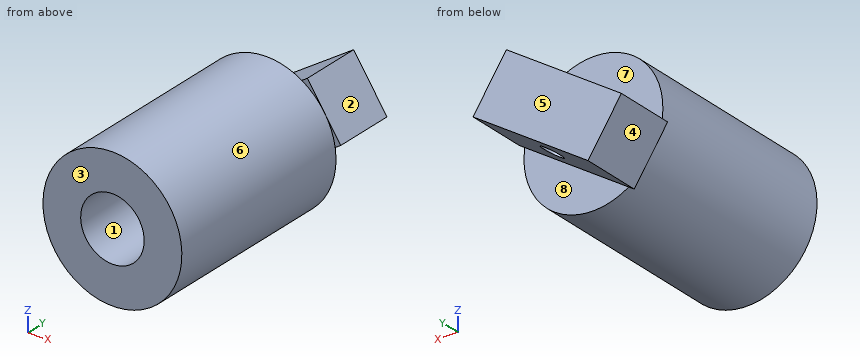
from build123d import *

# Parameters (mm, degrees)
SKETCH_1_R           = 3.5
EXTRUDE_2_DEPTH      = 10
SKETCH_2_R           = 1.6
CUT_EXTRUDE_1_DEPTH  = 7
EXTRUDE_4_DEPTH      = 1.5
EXTRUDE_4_DEPTH_BACK = 1.5
SKETCH_3_W           = 7
SKETCH_3_H           = 3
SKETCH_3_R           = 0.54827979


with BuildPart() as part:
    # Sketch 1 → Extrude 2 (new body)
    with BuildSketch(Plane(origin=(0, 0, 0), x_dir=(1, 0, 0), z_dir=(0, 1, 0))):
        with Locations(Location((0, 0, 0), (0, 0, 270))):
            Circle(SKETCH_1_R)
    extrude(amount=EXTRUDE_2_DEPTH)

    # Sketch 2 → Cut-Extrude 1 (cut)
    with BuildSketch(Plane.XZ):
        with Locations(Location((0, 0, 0), (0, 0, 270))):
            Circle(SKETCH_2_R)
    extrude(amount=-CUT_EXTRUDE_1_DEPTH, mode=Mode.SUBTRACT)

    # Sketch 3 → Extrude 4 (add, two sides: drawn at the far end of the back side and taken through both)
    with BuildSketch(Plane(origin=(0, 0, 0), x_dir=(0.8279714138688067, 0, 0.5607703075378451), z_dir=(-0.5607703075378451, 0, 0.8279714138688067)).offset(-EXTRUDE_4_DEPTH_BACK)):
        with Locations((0, 11.5)):
            Rectangle(SKETCH_3_W, SKETCH_3_H)
        with Locations((0, 11.597681641)):
            Circle(SKETCH_3_R, mode=Mode.SUBTRACT)
    extrude(amount=EXTRUDE_4_DEPTH + EXTRUDE_4_DEPTH_BACK)


solid = part.part
Verification items for the finished model (mm, model axes). Face numbers are marked on the shaded views. A direction names the side the tool comes from. Coordinates: 2 decimals unless noted, no trailing zeros. Write each loop counter-clockwise with the first axis right and the second up, starting at its lowest first coordinate (ties: lowest second). Pieces come first, ordered by that corner, then holes. Notation, with made-up numbers: (-7.75, 20.5) - (-1.75, 20.5) arc R33 cw to (-1.75, 53.5) - close; hole circle Ø7 at (-12, -26). An arc over 180 degrees is marked (long way). Answer as a JSON object with one key per item and string values.
(1) Cross-section at A-A on y = 2.25. Record the cut outline in (x, z), plus the area to 3 significant figures.
Report:
{"outline": "circle Ø7 at (0, 0); hole circle Ø3.2 at (0, 0)", "area": "30.4 mm^2"}
(2) Gauge pin test, flat ends, axial feed: pin 1 Ø3 at (x, y) = (-2, 8.5) entering from -Z; pin 2 Ø1 at (x, y) = (-2, 3.5) entering from +Z; pin 3 Ø3 at (x, z) = (0, 0) entering from -Y. Record the tip position at first contact, or that the pin passes through.
Report:
{"pin 1": "z = -3.46", "pin 2": "z = 3.16", "pin 3": "y = 7"}
(3) Tool access check on the marked faces 5, 6, 7 and 8. Record the directions out of +Z, -Z, +X, -X, +Y, -Y that give a thin tool (end or side, any length) a straight path to the whole face; none if there is none.
Report:
{"face 5": "+Z, -Z, +X, -X, +Y", "face 6": "-Y", "face 7": "+Z, -X, +Y", "face 8": "-Z, +X, +Y"}
(4) Cross-section at D-D on y = 8. Record the cut outline in (x, z).
Report:
{"outline": "circle Ø7 at (0, 0)"}
(5) Thickness scan on line 1 along X through (y, z) = (5.5, 0); line 2 along Y through (x, z) = (2, -2.25); line 3 along Z through (x, y) = (0.5, 2.5). Record the ranges inside material, lowest first.
Report:
{"line 1": "-3.5 to -1.6, 1.6 to 3.5", "line 2": "0 to 10", "line 3": "-3.46 to -1.52, 1.52 to 3.46"}
(6) Cross-section at B-B on x = -2.5. Record the cut outline in (y, z).
Report:
{"outline": "(0, -2.45) - (10, -2.45) - (10, -2.55) - (13, -2.55) - (13, 0.12) - (10, 0.12) - (10, 2.45) - (0, 2.45) - close"}
(7) Mould release check, pull along X, two halves, no side actions. Record for the marked faces 1, 2, 3 and 4: pulls with the +X half, pulls with the -X half, needs draft (parallel to the pull), parting line crosses it, or undercut.
Report:
{"face 1": "undercut", "face 2": "pulls with the +X half", "face 3": "needs draft", "face 4": "pulls with the -X half"}
